```python
from build123d import *

# Parameters (mm, degrees)
F0_R        = 11
F0_R_2      = 8.5
F1_DEPTH    = 40
F2_T        = -4
F3_DEPTH    = 2
F5_DEPTH    = 2
F7_DEPTH    = 2
F8_T1_DEPTH = 64


# Not quite as in the source:
# - a fillet or chamfer that OpenCascade refuses, or shapes differently, is made with other operations: its cross-section is extruded or revolved along the edge and cut away or added


with BuildPart() as f1:
    # F0 (on Right) → F1 (new body)
    with BuildSketch(Plane.YZ):
        with BuildLine():
            Line((63.6921661989, -31.096493093), (63.6921661989, 38.9364992437))
            Line((63.6921661989, 38.9364992437), (18.6921661989, 38.9364992437))
            Line((18.6921661989, 38.9364992437), (9.5297960554, 0))
            Line((9.5297960554, 0), (0, -10.2558757374))
            Line((0, -10.2558757374), (-12.9771592787, -17.7787300531))
            Line((-12.9771592787, -17.7787300531), (-43.6068768529, -22.555800424))
            Line((-43.6068768529, -22.555800424), (-58.6068768529, -22.555800424))
            ThreePointArc((-58.6068768529, -22.555800424), (-65.0535615803, -24.0913867663), (-70.115709102, -28.3683520288))
            Line((-70.115709102, -28.3683520288), (-51.312591107, -31.096493093))
            Line((-51.312591107, -31.096493093), (63.6921661989, -31.096493093))
        make_face()
        with Locations((47.8400811553, 10.7847582549)):
            Circle(F0_R, mode=Mode.SUBTRACT)
        Polygon((63.6921661989, -41.0635007563), (63.6921661989, -31.096493093), (-51.312591107, -31.096493093), (-70.115709102, -28.3683520288), (-70.115709102, -38.3683520288), (-51.3078338011, -41.0635007563), align=None)
        with Locations((47.8400811553, 10.7847582549)):
            Circle(F0_R)
        with Locations((47.8400811553, 10.7847582549)):
            Circle(F0_R_2, mode=Mode.SUBTRACT)
        with Locations((47.8400811553, 10.7847582549)):
            Circle(F0_R_2)
    extrude(amount=F1_DEPTH)

    # F2
    f2_openings = [f1.faces().sort_by_distance(p)[0] for p in [
        (20, 41.192166, 38.936499),
    ]]
    offset(amount=F2_T, openings=f2_openings, kind=Kind.INTERSECTION)

    # F3 (add): a face of the model
    f3_faces = [f1.faces().sort_by_distance(p)[0] for p in [
        (20, -70.115709102, -33.3683520288),
    ]]
    extrude(f3_faces, amount=F3_DEPTH)

    # F4 (on face) → F5 (join)
    with BuildSketch(Plane.YZ.offset(40)):
        Polygon((63.6921661989, -28.3683520288), (-70.115709102, -28.3683520288), (-72.115709102, -28.3683520288), (-72.115709102, -38.3683520288), (-70.115709102, -38.3683520288), (-51.3078338011, -41.0635007563), (63.6921661989, -41.0635007563), align=None)
    extrude(amount=F5_DEPTH)

    # F6 (on face) → F7 (join)
    with BuildSketch(Plane(origin=(0, 0, 0), x_dir=(0, -1, 0), z_dir=(-1, 0, 0))):
        Polygon((72.115709102, -28.3683520288), (70.115709102, -28.3683520288), (-63.6921661989, -28.3683520288), (-63.6921661989, -41.0635007563), (51.3078338011, -41.0635007563), (70.115709102, -38.3683520288), (72.115709102, -38.3683520288), align=None)
    extrude(amount=F7_DEPTH)

    # F8: fillet of radius 5 on 1 edges, made by hand

    # F8_s2 → F8_t1 (cut)
    with BuildSketch(Plane.YZ.offset(-12)):
        with BuildLine():
            ThreePointArc((-70.115709102, -38.3683520288), (-71.587845057, -36.6044200063), (-72.115709102, -34.3683520288))
            Line((-72.115709102, -34.3683520288), (-72.115709102, -38.3683520288))
            Line((-72.115709102, -38.3683520288), (-70.115709102, -38.3683520288))
        make_face()
    extrude(amount=F8_T1_DEPTH, mode=Mode.SUBTRACT)


solid = f1.part
```
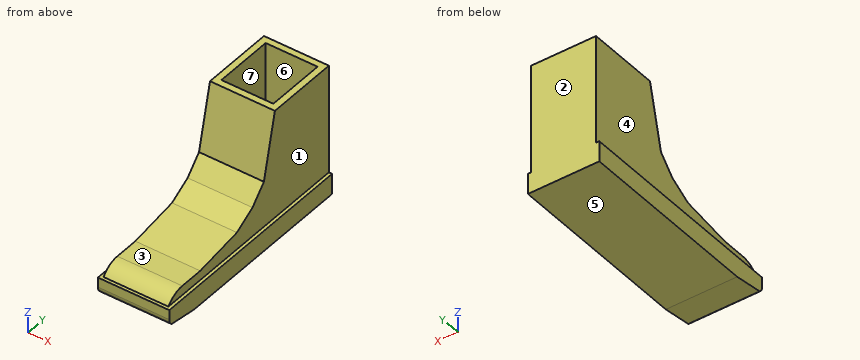
Could you check a few things on this model? Use its own coordinates, in mm. Face numbers are marked on the shaded views. A direction names the side the tool comes from. Round coordinates to 2 decimals unless told otherwise and drop trailing zeros. Loops run counter-clockwise (first coordinate to the right, second up) from the corner with the lowest first, then second, coordinate; pieces in that order, holes last. Notation, with made-up numbers: (1, 23.5) -> (57, 23.5) arc R17 ccw to (57, 45.5) -> close; hole circle Ø8 at (-18.75, -33). An arc over 180 degrees is marked (long way). One line per question, with ' | ' between items.
(1) If I drill on probe 1 along X at (y, z) = (42.5, 5); probe 2 along Y at (x, z) = (13.5, -32); probe 3 along Z at (x, y) = (21.5, 46.5), over which ranges is the centre line in solid material (lowest first)?
Model answer:
probe 1: x = 0 to 4, 36 to 40 | probe 2: y = -72.12 to -66.12, 59.69 to 63.69 | probe 3: z = -41.06 to -37.06
(2) If we section it at D-D on y = 36.5: List the corners of the cut face in (x, z) for me.
Model answer:
outline: (-2, -41.06) -> (42, -41.06) -> (42, -28.37) -> (40, -28.37) -> (40, 38.94) -> (36, 38.94) -> (36, -37.06) -> (4, -37.06) -> (4, 38.94) -> (0, 38.94) -> (0, -28.37) -> (-2, -28.37) -> close
(3) For the marked faces 1, 2, 3 and 4, which set-ups out of +Z, -Z, +X, -X, +Y, -Y let a thin tool reach every point of the face, with its end or its side?
Model answer:
face 1: +Z, +X, +Y, -Y | face 2: +Z, -Z, +X, -X, +Y | face 3: +Z, +X, -X, -Y | face 4: +Z, -X, +Y, -Y
(4) If we section it at C-C on x = 18: List the corners of the cut face in (y, z) for me, and give its area (3 significant figures).
Model answer:
outline: (-72.12, -34.37) arc R5 ccw to (-70.12, -38.37) -> (-51.31, -41.06) -> (63.69, -41.06) -> (63.69, 38.94) -> (59.69, 38.94) -> (59.69, -37.06) -> (-51.02, -37.06) -> (-66.12, -34.9) -> (-66.12, -29.81) arc R10.3 cw to (-58.61, -26.56) -> (-43.3, -26.56) -> (-11.62, -21.62) -> (2.52, -13.42) -> (13.18, -1.95) -> (22.8, 38.94) -> (18.69, 38.94) -> (9.53, 0) -> (0, -10.26) -> (-12.98, -17.78) -> (-43.61, -22.56) -> (-58.61, -22.56) arc R14.3 ccw to (-70.12, -28.37) -> (-72.12, -28.37) -> close | area: 1,400 mm^2
(5) If we section it at A-A on z = -32: List the corners of the cut face in (x, y) for me, and give its area (3 significant figures).
Model answer:
outline: (-2, -72.12) -> (42, -72.12) -> (42, 63.69) -> (-2, 63.69) -> close; hole (4, -66.12) -> (36, -66.12) -> (36, 59.69) -> (4, 59.69) -> close | area: 1,950 mm^2
(6) Thinking about a two-plate mould opening in Z: for the marked faces 5, 6 and 7, which applies, released by +Z, released by -Z, zero draft, split by the parting line, or undercut?
Model answer:
face 5: released by -Z | face 6: zero draft | face 7: undercut
(7) If we section it at B-B on y = -49: List the corners of the cut face in (x, z) for me.
Model answer:
outline: (-2, -41.06) -> (42, -41.06) -> (42, -28.37) -> (40, -28.37) -> (40, -22.56) -> (0, -22.56) -> (0, -28.37) -> (-2, -28.37) -> close; hole (4, -37.06) -> (36, -37.06) -> (36, -26.56) -> (4, -26.56) -> close
(8) For pin 1 Ø12 at (x, y) = (30, -53) entering from +Z; pin 2 Ø16 at (x, z) = (22, 5) entering from -Y; pin 3 Ø8 at (x, z) = (30.5, 22.5) entering from -Y, each with a flat end and sliding along its axis, tell me the tip position at first contact or that it passes through.
Model answer:
pin 1: stops at z = -22.56 | pin 2: stops at y = 6.74 | pin 3: stops at y = 13.88
